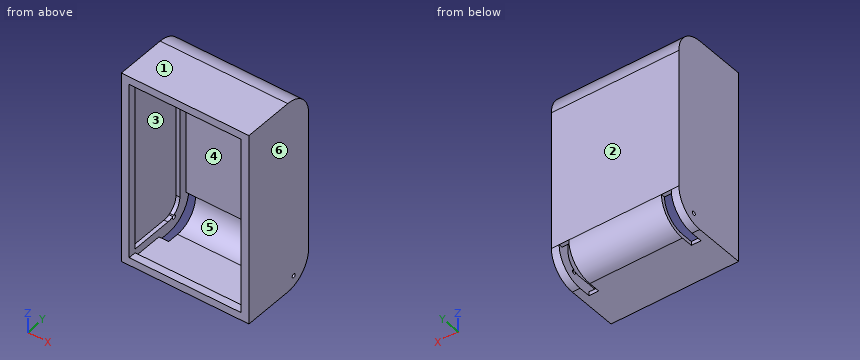
from build123d import *

# Parameters (mm, degrees)
F0_W      = 330
F0_H      = 500
F1_DEPTH  = 200
F2_R      = 70
F3_T      = -10
F5_DEPTH  = 10
F7_DEPTH  = 10
F8_W      = 290
F8_H      = 20
F9_DEPTH  = 10
F10_W     = 290
F10_H     = 20
F11_DEPTH = 10
F13_W     = 25
F13_H     = 100
F14_DEPTH = 70
F15_R     = 5
F16_DEPTH = 330.001


with BuildPart() as f1:
    # F0 (on Front) → F1 (new body)
    with BuildSketch(Plane.XZ):
        with Locations((165, -250)):
            Rectangle(F0_W, F0_H)
    extrude(amount=-F1_DEPTH)

    # F2
    f2_edges = [f1.edges().sort_by_distance(p)[0] for p in [
        (165, 200, 0),
        (165, 200, -500),
    ]]
    fillet(f2_edges, radius=F2_R)

    # F3
    f3_openings = [f1.faces().sort_by_distance(p)[0] for p in [
        (165, 0, -250),
    ]]
    offset(amount=F3_T, openings=f3_openings)

    # F4 (on face) → F5 (join)
    with BuildSketch(Plane.YZ.offset(10)):
        with BuildLine():
            ThreePointArc((190, -70), (172.426407, -27.573593), (130, -10))
            Line((130, -10), (0, -10))
            Line((0, -10), (0, -490))
            Line((0, -490), (130, -490))
            ThreePointArc((130, -490), (172.426407, -472.426407), (190, -430))
            Line((190, -430), (190, -70))
        make_face()
        with BuildLine():
            ThreePointArc((170, -430), (158.284271, -458.284271), (130, -470))
            Line((130, -470), (20, -470))
            Line((20, -470), (20, -30))
            Line((20, -30), (130, -30))
            ThreePointArc((130, -30), (158.284271, -41.715729), (170, -70))
            Line((170, -70), (170, -430))
        make_face(mode=Mode.SUBTRACT)
    extrude(amount=F5_DEPTH)

    # F6 (on face) → F7 (join)
    with BuildSketch(Plane(origin=(320, 0, 0), x_dir=(0, -1, 0), z_dir=(-1, 0, 0))):
        with BuildLine():
            ThreePointArc((-190, -430), (-172.426407, -472.426407), (-130, -490))
            Line((-130, -490), (0, -490))
            Line((0, -490), (0, -10))
            Line((0, -10), (-130, -10))
            ThreePointArc((-130, -10), (-172.426407, -27.573593), (-190, -70))
            Line((-190, -70), (-190, -430))
        make_face()
        with BuildLine():
            Line((-20, -470), (-130, -470))
            ThreePointArc((-130, -470), (-158.284271, -458.284271), (-170, -430))
            Line((-170, -430), (-170, -70))
            ThreePointArc((-170, -70), (-158.284271, -41.715729), (-130, -30))
            Line((-130, -30), (-20, -30))
            Line((-20, -30), (-20, -470))
        make_face(mode=Mode.SUBTRACT)
    extrude(amount=F7_DEPTH)

    # F8 (on face) → F9 (join)
    with BuildSketch(Plane.XY.offset(-490)):
        with Locations((165, 10)):
            Rectangle(F8_W, F8_H)
    extrude(amount=F9_DEPTH)

    # F10 (on face) → F11 (join)
    with BuildSketch(Plane(origin=(0, 0, -10), x_dir=(1, 0, 0), z_dir=(0, 0, -1))):
        with Locations((165, -10)):
            Rectangle(F10_W, F10_H)
    extrude(amount=F11_DEPTH)

    # F13 (on face) → F14 (cut)
    with BuildSketch(Plane(origin=(0, 0, -500), x_dir=(1, 0, 0), z_dir=(0, 0, -1))):
        with Locations((32.5, -150)):
            Rectangle(F13_W, F13_H)
        with Locations((297.5, -150)):
            Rectangle(F13_W, F13_H)
    extrude(amount=-F14_DEPTH, mode=Mode.SUBTRACT)

    # F15 (on face) → F16 (cut, through all)
    with BuildSketch(Plane(origin=(0, 0, 0), x_dir=(0, -1, 0), z_dir=(-1, 0, 0))):
        with Locations((-150, -470)):
            Circle(F15_R)
    extrude(amount=-F16_DEPTH, mode=Mode.SUBTRACT)


solid = f1.part
Input: part model. Units: mm. Frame: model coordinates. Face numbers are marked on the shaded views. A direction names the side the tool comes from. Give positions to 0.01 mm unless a question says otherwise; leave off trailing zeros. Order: outer loops, then holes, each group sorted by start corner. A loop starts at its lowest first (then second) coordinate and runs counter-clockwise, first axis right, second up. Notation, with made-up numbers: (-33, -40) - (16, -40) arc R9 cw to (16, -25) - close; hole circle Ø3 at (80, 58). An arc over 180 degrees is marked (long way). Write each question's results on one line, items separated by ' | '.
Item 1: Section A-A (y = 14.5). Return loops of the section in (x, z), and give its area (3 significant figures).
A:
outline: (0, -500) - (330, -500) - (330, 0) - (0, 0) - close; hole (20, -480) - (310, -480) - (310, -20) - (20, -20) - close | area: 31,600 mm^2
Item 2: Section D-D (y = 89.5). Return loops of the section in (x, z).
A:
outline: (0, -500) - (330, -500) - (330, 0) - (0, 0) - close; hole (10, -470) - (20, -470) - (20, -490) - (310, -490) - (310, -470) - (320, -470) - (320, -30) - (310, -30) - (310, -10) - (20, -10) - (20, -30) - (10, -30) - close
Item 3: Access query for the marked faces 4, 5 and 6. Directions: +Z, -Z, +X, -X, +Y, -Y. A direction counts if a zero-diameter tool reaches every point of the face in a straight line with its end or side. Return the directions, or none.
A:
face 4: -Y | face 5: none | face 6: +Z, -Z, +X, +Y, -Y
Item 4: Contact query for flat-ended pins moving along their axis: pin 1 Ø6 at (x, z) = (110.5, -63.5) entering from -Y; pin 2 Ø3 at (x, y) = (98.5, 172.5) entering from +Z; pin 3 Ø3 at (x, y) = (37.5, 193.5) entering from -Z. Output: stop coordinate, or through.
A:
pin 1: stops at y = 189.24 | pin 2: stops at z = -13.26 | pin 3: stops at z = -430
Item 5: Section C-C (x = 105.5). Return loops of the section in (y, z), and give its area (3 significant figures).
A:
outline: (0, -500) - (130, -500) arc R70 ccw to (200, -430) - (200, -70) arc R70 ccw to (130, 0) - (0, 0) - (0, -20) - (20, -20) - (20, -10) - (130, -10) arc R60 cw to (190, -70) - (190, -430) arc R60 cw to (130, -490) - (20, -490) - (20, -480) - (0, -480) - close | area: 8,640 mm^2
Item 6: Material intervals for line 1 along X through (y, z) = (35.5, -292); line 2 along Z through (x, y) = (39, 73); line 3 along X through (y, z) = (11, -420), sorted ascending.
A:
line 1: x = 0 to 10, 320 to 330 | line 2: z = -500 to -490, -10 to 0 | line 3: x = 0 to 20, 310 to 330
Item 7: Section B-B (z = -377). Return loops of the section in (x, y), and give its area (3 significant figures).
A:
outline: (0, 0) - (20, 0) - (20, 20) - (10, 20) - (10, 170) - (20, 170) - (20, 190) - (310, 190) - (310, 170) - (320, 170) - (320, 20) - (310, 20) - (310, 0) - (330, 0) - (330, 200) - (0, 200) - close | area: 7,900 mm^2
Item 8: Draft query along Y for the marked faces 1, 2 and 3. Return one class per face: released by +Y, released by -Y, zero draft, split by the parting line, or undercut.
A:
face 1: zero draft | face 2: released by +Y | face 3: undercut
